Autodesk Inventor part; units mm, degrees
ref_plane "YZ Plane" through (0, 0, 0) normal (1, 0, 0) x (0, 1, 0)
ref_plane "XZ Plane" through (0, 0, 0) normal (0, 1, 0) x (-1, 0, 0)
ref_plane "XY Plane" through (0, 0, 0) normal (0, 0, 1) x (1, 0, 0)
sketch "Sketch1" plane through (0, 0, 0) normal (0, 0, 1) x (1, 0, 0)
  line L0 (0, 9.5) -> (-3, 9.5)
  line L1 (-3, 9.5) -> (-3, 15.5)
  line L2 (-3, 15.5) -> (0, 15.5)
  line L3 (0, 15.5) -> (0, 25)
  line L4 (44, 25) -> (44, 15.5)
  line L5 (44, 15.5) -> (47, 15.5)
  line L6 (47, 15.5) -> (47, 9.5)
  line L7 (47, 9.5) -> (44, 9.5)
  line L8 (44, 9.5) -> (44, 0)
  line L9 (0, 0) -> (0, 9.5)
  line L10 (0, 25) -> (17, 25)
  line L11 (17, 25) -> (17, 28)
  line L12 (17, 28) -> (27, 28)
  line L13 (27, 28) -> (27, 25)
  line L14 (27, 25) -> (44, 25)
  line L15 (0, 0) -> (17, 0)
  line L16 (17, 0) -> (17, -3)
  line L17 (17, -3) -> (27, -3)
  line L18 (27, -3) -> (27, 0)
  line L19 (27, 0) -> (44, 0)
  dimension "d0" = 6
  dimension "d1" = 3
  dimension "d2" = 3
  dimension "d3" = 6
  dimension "d4" = 50
  dimension "d5" = 3
  dimension "d6" = 10
  dimension "d7" = 3
  dimension "d14" = 25
extrude "Extrusion1" add sketch "Sketch1" along normal blind 3
Geometry check sheet. Reference: the model listing, model coordinates, mm. A direction names the side the tool comes from. Give positions to 0.01 mm unless a question says otherwise; leave off trailing zeros. Order: outer loops, then holes, each group sorted by start corner. A loop starts at its lowest first (then second) coordinate and runs counter-clockwise, first axis right, second up.
1) Cross-section at A-A (z = 1.3). Record the boundary of the cut face in (x, y), then the cut area to 3 significant figures.
Results are:
outline: (-3, 9.5) - (0, 9.5) - (0, 0) - (17, 0) - (17, -3) - (27, -3) - (27, 0) - (44, 0) - (44, 9.5) - (47, 9.5) - (47, 15.5) - (44, 15.5) - (44, 25) - (27, 25) - (27, 28) - (17, 28) - (17, 25) - (0, 25) - (0, 15.5) - (-3, 15.5) - close
area: 1,200 mm2
2) Gauge pin test, flat ends, axial feed: pin 1 (1 mm diameter, centred on x = 33.5, y = 4.5, fed in from -Z); pin 2 (1.5 mm diameter, centred on y = 20.5, z = 1, fed in from -X); pin 3 (1.5 mm diameter, centred on x = 38.5, z = 1.5, fed in from +Y); pin 4 (1.5 mm diameter, centred on y = 4.5, z = 1, fed in from +X). Record the tip position at first contact, or that the pin passes through.
Results are:
pin 1: stops at z = 0
pin 2: stops at x = 0
pin 3: stops at y = 25
pin 4: stops at x = 44
3) Tool access check on faces 1 (the flat face through (17, 26, 1)), 2 (the flat face through (17, -1, 1)), 3 (the flat face through (27, -2, 1)), 4 (the flat face through (44, 20, 1)). Record the directions out of +Z, -Z, +X, -X, +Y, -Y that give a thin tool (end or side, any length) a straight path to the whole face; none if there is none.
Results are:
face 1: +Z, -Z, -X, +Y
face 2: +Z, -Z, -X, -Y
face 3: +Z, -Z, +X, -Y
face 4: +Z, -Z, +X, +Y
4) Cross-section at B-B (x = 30). Record the boundary of the cut face in (y, z), then the cut area to 3 significant figures.
Results are:
outline: (0, 0) - (25, 0) - (25, 3) - (0, 3) - close
area: 75.0 mm2
5) Cross-section at C-C (y = 1.5). Record the boundary of the cut face in (x, z).
Results are:
outline: (0, 0) - (44, 0) - (44, 3) - (0, 3) - close
6) Material ranges on probe 1 along Y at (x, z) = (36, 2.25); probe 2 along X at (y, z) = (20.5, 1.65); probe 3 along X at (y, z) = (27.5, 0.7), recorded low to high.
Results are:
probe 1: y = 0 to 25
probe 2: x = 0 to 44
probe 3: x = 17 to 27
